Read the model definition and answer for the solid it produces. Units are mm, in the model's axes. A direction names the side the tool comes from. Give positions to 0.01 mm unless a question says otherwise; leave off trailing zeros. Order: outer loops, then holes, each group sorted by start corner. A loop starts at its lowest first (then second) coordinate and runs counter-clockwise, first axis right, second up. Notation, with made-up numbers: (10.5, 1.5) -> (16.5, 1.5) arc R26 ccw to (16.5, 25.5) -> close; hole circle Ø11 at (-6, -29). An arc over 180 degrees is marked (long way). Answer as CSV lines item,"result". Start each with the question number.
1) Straight lines are drawn through the part: L1, parallel to Y at x = -20, z = 3; L2, parallel to Y at x = -29, z = 4.35; L3, parallel to X at y = 10, z = 2.9. For each, find the intervals that lie inside material, in ascending order. Write a range as from..to.
2) The mould has two halves that part along X. Classify faces 1 (the face through (-30, 45, 2)), 2 (the face through (-35, 40, 2)), 3 (the face through (-5, 38, 2)): +X half, -X half, draft (parallel to the pull), parting line (faces both ways), or undercut.
3) Find section A-A (x = -20). Determine the outline of the cut face in (y, z).
4) A flat-ended cylindrical pin translates along its axis: pin 1 Ø2.5 at (y, z) = (41, 1.5) entering from +X. Find the tip coordinate at first contact, or state that the pin passes through.
5) Find section B-B (y = 15). Determine the outline of the cut face in (x, z).
6) Find section D-D (z = 1.5). Determine the outline of the cut face in (x, y).
7) For faces 4 (the face through (-5, -7, 2)), 5 (the face through (-27, 15, 0)), 6 (the face through (-43, 25, 2)), 7 (the face through (-3, 30, 2)), determine the directions among +Z, -Z, +X, -X, +Y, -Y from which every point of the face is accessible in a straight line to the end or side of a thin tool.
8) Find section C-C (y = 21). Determine the outline of the cut face in (x, z).
```python
from build123d import *

# Parameters (mm, degrees)
ESQUISSE1_R        = 2
ESQUISSE1_W        = 20
ESQUISSE1_H        = 5
ESQUISSE1_W_2      = 5
ESQUISSE1_H_2      = 20
BOSS_EXTRU_1_DEPTH = 5


with BuildPart() as part:
    # Esquisse1 → Boss.-Extru.1 (new body)
    with BuildSketch(Plane.XY):
        Polygon((-55, 45), (-5, 45), (-5, 30), (0, 30), (0, 0), (-5, 0), (-5, -15), (-55, -15), align=None)
        with Locations((-20, 30)):
            Circle(ESQUISSE1_R, mode=Mode.SUBTRACT)
        with Locations((-20, 15)):
            Circle(ESQUISSE1_R, mode=Mode.SUBTRACT)
        with Locations((-35, 37.5)):
            Rectangle(ESQUISSE1_W, ESQUISSE1_H, mode=Mode.SUBTRACT)
        with Locations((-42.5, 15)):
            Rectangle(ESQUISSE1_W_2, ESQUISSE1_H_2, mode=Mode.SUBTRACT)
    extrude(amount=BOSS_EXTRU_1_DEPTH)


solid = part.part
```
Findings below:
1,L1,"-15..13, 17..28, 32..45"
1,L2,"-15..35, 40..45"
1,L3,"-55..-45, -40..0"
2,face 1,"draft"
2,face 2,"undercut"
2,face 3,"+X half"
3,outline,"(-15, 0) -> (13, 0) -> (13, 5) -> (-15, 5) -> close; (17, 0) -> (28, 0) -> (28, 5) -> (17, 5) -> close; (32, 0) -> (45, 0) -> (45, 5) -> (32, 5) -> close"
4,pin 1,"x = -5"
5,outline,"(-55, 0) -> (-45, 0) -> (-45, 5) -> (-55, 5) -> close; (-40, 0) -> (-22, 0) -> (-22, 5) -> (-40, 5) -> close; (-18, 0) -> (0, 0) -> (0, 5) -> (-18, 5) -> close"
6,outline,"(-55, -15) -> (-5, -15) -> (-5, 0) -> (0, 0) -> (0, 30) -> (-5, 30) -> (-5, 45) -> (-55, 45) -> close; hole (-45, 5) -> (-40, 5) -> (-40, 25) -> (-45, 25) -> close; hole (-45, 35) -> (-25, 35) -> (-25, 40) -> (-45, 40) -> close; hole circle Ø4 at (-20, 15); hole circle Ø4 at (-20, 30)"
7,face 4,"+Z, -Z, +X, -Y"
7,face 5,"-Z, +X, -X, +Y, -Y"
7,face 6,"+Z, -Z"
7,face 7,"+Z, -Z, +X, +Y"
8,outline,"(-55, 0) -> (-45, 0) -> (-45, 5) -> (-55, 5) -> close; (-40, 0) -> (0, 0) -> (0, 5) -> (-40, 5) -> close"
